```python
from build123d import *

# Parameters (mm, degrees)
EXTRUDE_2_DEPTH     = 10
SKETCH_8_R          = 1.8
CUT_EXTRUDE_3_DEPTH = 5
SKETCH_9_W          = 5.8
SKETCH_9_H          = 5.8
CUT_EXTRUDE_4_DEPTH = 14


with BuildPart() as part:
    # 草图1 → 凸台-拉伸2 (new body)
    with BuildSketch(Plane(origin=(0, 0, 0), x_dir=(1, 0, 0), z_dir=(0, 1, 0))):
        with BuildLine():
            Line((-69.33427814, 6.574466706), (-56.33427814, 6.574466706))
            ThreePointArc((-56.33427814, 6.574466706), (-40.33427814, 22.574466706), (-24.33427814, 6.574466706))
            Line((-24.33427814, 6.574466706), (-11.33427814, 6.574466706))
            Line((-11.33427814, 6.574466706), (-11.33427814, 25.574466706))
            Line((-11.33427814, 25.574466706), (-69.33427814, 25.574466706))
            Line((-69.33427814, 25.574466706), (-69.33427814, 6.574466706))
        make_face()
    extrude(amount=EXTRUDE_2_DEPTH)

    # 草图8 → 切除-拉伸3 (cut)
    with BuildSketch(Plane.XY.offset(-6.574466706)):
        with Locations((-62.83427814, 5)):
            Circle(SKETCH_8_R)
        with Locations((-17.83427814, 5)):
            Circle(SKETCH_8_R)
    extrude(amount=-CUT_EXTRUDE_3_DEPTH, mode=Mode.SUBTRACT)

    # 草图9 → 切除-拉伸4 (cut)
    with BuildSketch(Plane(origin=(0, 0, -25.574466706), x_dir=(-1, 0, 0), z_dir=(0, 0, -1))):
        with Locations((17.83427814, 5)):
            Rectangle(SKETCH_9_W, SKETCH_9_H)
        with Locations((62.83427814, 5)):
            Rectangle(SKETCH_9_W, SKETCH_9_H)
    extrude(amount=-CUT_EXTRUDE_4_DEPTH, mode=Mode.SUBTRACT)


solid = part.part
```
Could you check a few things on this model? Use its own coordinates, in mm. A direction names the side the tool comes from. Round coordinates to 2 decimals unless told otherwise and drop trailing zeros. Order: outer loops, then holes, each group sorted by start corner. A loop starts at its lowest first (then second) coordinate and runs counter-clockwise, first axis right, second up. Notation, with made-up numbers: M 79,-38.5 L 117,-38.5 A12 ccw 117,-29.5 Z; hole C 23,20 d1. An arc over 180 degrees is marked long. One line per question, with ' | ' between items. Start each with the question number.
(1) For P1, Ø2, axis at x = -62.83, y = 5, coming from the -Z side; P2, Ø3, axis at x = -62, y = 5.5, coming from the -Z side, each with a flat end and sliding along its axis, tell me the tip position at first contact or that it passes through.
(2) Suppose I cut it at C-C on x = -60.5. List the corners of the cut face in (y, z) for me.
(3) Please list where these lines run through material, in increasing order: line 1 along X through (y, z) = (7.5, -24); line 2 along Y through (x, z) = (-16, -24.25); line 3 along X through (y, z) = (6.75, -12).
(4) For faces 5 (the face through (-19.4, 3.8, -6.574)), 6 (the face through (-15.86, 5.04, -11.574)), which set-ups out of +Z, -Z, +X, -X, +Y, -Y let a thin tool reach every point of the face, with its end or its side?
(5) Thinking about a two-plate mould opening in X: for faces 1 (the face through (-63, 7.9, -19)), 2 (the face through (-41, 10, -25)), 3 (the face through (-11.334, 5, -16)), 4 (the face through (-18, 2.1, -19)), which applies, +X half, -X half, draft (parallel to the pull), parting line (faces both ways), or undercut?
(6) Suppose I cut it at D-D on z = -17.75. List the corners of the cut face in (x, y) for me.
(7) Suppose I cut it at A-A on z = -13. List the corners of the cut face in (x, y) for me.
(8) Suppose I cut it at B-B on y = 5. List the corners of the cut face in (x, z) for me.
Geometry results:
1) P1: through | P2: z = -11.57
2) outline: M 0,-25.57 L 2.1,-25.57 L 2.1,-11.57 L 7.9,-11.57 L 7.9,-25.57 L 10,-25.57 L 10,-6.57 L 0,-6.57 Z
3) line 1: -69.33 to -65.73, -59.93 to -20.73, -14.93 to -11.33 | line 2: 0 to 2.1, 7.9 to 10 | line 3: -69.33 to -65.73, -59.93 to -55.39, -25.28 to -20.73, -14.93 to -11.33
4) face 5: +Z, +X, -X, +Y, -Y | face 6: -Z
5) face 1: undercut | face 2: draft | face 3: +X half | face 4: undercut
6) outline: M -69.33,0 L -51.78,0 L -51.78,10 L -69.33,10 Z; M -28.88,0 L -11.33,0 L -11.33,10 L -28.88,10 Z; hole M -65.73,2.1 L -59.93,2.1 L -59.93,7.9 L -65.73,7.9 Z; hole M -20.73,2.1 L -14.93,2.1 L -14.93,7.9 L -20.73,7.9 Z
7) outline: M -69.33,0 L -54.99,0 L -54.99,10 L -69.33,10 Z; M -25.68,0 L -11.33,0 L -11.33,10 L -25.68,10 Z; hole M -65.73,2.1 L -59.93,2.1 L -59.93,7.9 L -65.73,7.9 Z; hole M -20.73,2.1 L -14.93,2.1 L -14.93,7.9 L -20.73,7.9 Z
8) outline: M -69.33,-25.57 L -65.73,-25.57 L -65.73,-11.57 L -64.63,-11.57 L -64.63,-6.57 L -69.33,-6.57 Z; M -61.03,-11.57 L -59.93,-11.57 L -59.93,-25.57 L -20.73,-25.57 L -20.73,-11.57 L -19.63,-11.57 L -19.63,-6.57 L -24.33,-6.57 A16 cw -56.33,-6.57 L -61.03,-6.57 Z; M -16.03,-11.57 L -14.93,-11.57 L -14.93,-25.57 L -11.33,-25.57 L -11.33,-6.57 L -16.03,-6.57 Z
